Geometry: final body of the model. Coordinates: model frame, mm. Face numbers are marked on the shaded views. A direction names the side the tool comes from. Coordinates: 2 decimals unless noted, no trailing zeros. Loops run counter-clockwise (first coordinate to the right, second up) from the corner with the lowest first, then second, coordinate; pieces in that order, holes last. Notation, with made-up numbers: M 4.5,28 L 28.5,28 A32 ccw 28.5,55 Z; hole C 77,-28 d8. An arc over 180 degrees is marked long. Write each question's results on one line, items separated by ' | '. Start each with the question number.
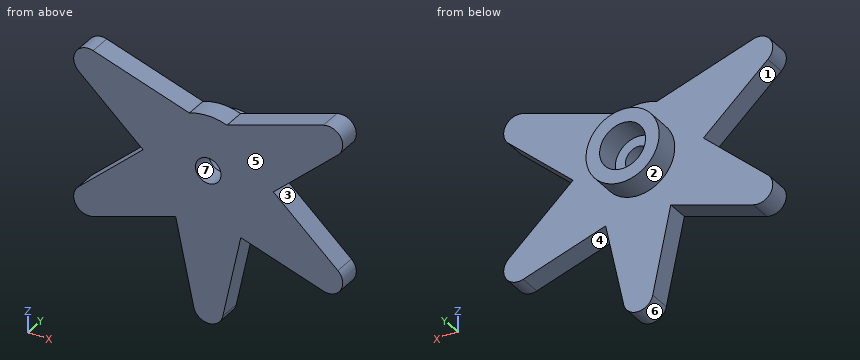
from build123d import *

# Parameters (mm, degrees)
SKETCH1_R           = 1.5
BOSS_EXTRUDE1_DEPTH = 2.6
SKETCH2_R           = 4.3
SKETCH2_R_2         = 2.7
BOSS_EXTRUDE2_DEPTH = 3


with BuildPart() as part:
    # Sketch1 → Boss-Extrude1 (new body)
    with BuildSketch(Plane(origin=(0, 0, 0), x_dir=(1, 0, 0), z_dir=(0, 1, 0))):
        with BuildLine():
            Line((3.832260045, 6.637669106), (1.711758301, 16.613845459))
            ThreePointArc((1.711758301, 16.613845459), (0, 18), (-1.711758301, 16.613845459))
            Line((-1.711758301, 16.613845459), (-3.832260045, 6.637669106))
            Line((-3.832260045, 6.637669106), (-13.532133071, 9.789348904))
            ThreePointArc((-13.532133071, 9.789348904), (-15.588457268, 9), (-15.243891373, 6.824496555))
            Line((-15.243891373, 6.824496555), (-7.664520091, 0))
            Line((-7.664520091, 0), (-15.243891373, -6.824496555))
            ThreePointArc((-15.243891373, -6.824496555), (-15.588457268, -9), (-13.532133071, -9.789348904))
            Line((-13.532133071, -9.789348904), (-2.213204152, -6.111605957))
            ThreePointArc((-2.213204152, -6.111605957), (0, -6.5), (2.213204152, -6.111605957))
            Line((2.213204152, -6.111605957), (13.532133071, -9.789348904))
            ThreePointArc((13.532133071, -9.789348904), (15.588457268, -9), (15.243891373, -6.824496555))
            Line((15.243891373, -6.824496555), (7.664520091, 0))
            Line((7.664520091, 0), (15.243891373, 6.824496555))
            ThreePointArc((15.243891373, 6.824496555), (15.588457268, 9), (13.532133071, 9.789348904))
            Line((13.532133071, 9.789348904), (3.832260045, 6.637669106))
        make_face()
        with Locations(Location((0, 0, 0), (0, 0, 270))):
            Circle(SKETCH1_R, mode=Mode.SUBTRACT)
    extrude(amount=BOSS_EXTRUDE1_DEPTH)

    # Sketch2 → Boss-Extrude2 (add)
    with BuildSketch(Plane(origin=(0, 2.6, 0), x_dir=(1, 0, 0), z_dir=(0, 1, 0))):
        with Locations(Location((0, 0, 0), (0, 0, 270))):
            Circle(SKETCH2_R)
        with Locations(Location((0, 0, 0), (0, 0, 270))):
            Circle(SKETCH2_R_2, mode=Mode.SUBTRACT)
    extrude(amount=BOSS_EXTRUDE2_DEPTH)


solid = part.part
Item 1: Set-up query: the marked faces 1, 2, 3 and 4. Return all of +Z, -Z, +X, -X, +Y, -Y with unobstructed straight access to the full face (end or side cutting, diameter ignored); none if empty.
Item 2: Section D-D, the plane y = 3.15. Return loops of the section in (x, z).
Item 3: Ray query, L1, parallel to X at y = 4.4, z = 0; L2, parallel to Y at x = 9.5, z = 5.25; L3, parallel to X at y = 1.45, z = -1. Return the intervals inside material, ascending. Write a range as [from, to].
Item 4: Contact query for a flat-ended pin moving along its axis: P1, Ø2.5, axis at x = 0.5, z = -0.5, coming from the +Y side. Output: stop coordinate, or through.
Item 5: Pull-direction query (X, two-part tool) for the marked faces 5, 6 and 7; classes: released by +X, released by -X, zero draft, split by the parting line, or undercut.
Item 6: Section B-B, the plane x = 0. Return loops of the section in (y, z), plus the area to 3 significant figures.
Item 7: Section C-C, the plane z = -1. Return loops of the section in (x, y), plus the area to 3 significant figures.
Solutions:
1) face 1: -X, +Y, -Y | face 2: +Y | face 3: +X, +Y, -Y | face 4: -Z, +Y, -Y
2) outline: C 0,0 d8.6; hole C 0,0 d5.4
3) L1: x = [-4.3, -2.7], [2.7, 4.3] | L2: y = [0, 2.6] | L3: x = [-8.78, -1.12], [1.12, 8.78]
4) P1: stops at y = 2.6
5) face 5: zero draft | face 6: split by the parting line | face 7: undercut
6) outline: M 0,-18 L 2.6,-18 L 2.6,-4.3 L 5.6,-4.3 L 5.6,-2.7 L 2.6,-2.7 L 2.6,-1.5 L 0,-1.5 Z; M 0,1.5 L 2.6,1.5 L 2.6,2.7 L 5.6,2.7 L 5.6,4.3 L 2.6,4.3 L 2.6,6.5 L 0,6.5 Z | area: 65.5 mm²
7) outline: M -8.78,0 L -1.12,0 L -1.12,2.6 L -2.51,2.6 L -2.51,5.6 L -4.18,5.6 L -4.18,2.6 L -8.78,2.6 Z; M 1.12,0 L 8.78,0 L 8.78,2.6 L 4.18,2.6 L 4.18,5.6 L 2.51,5.6 L 2.51,2.6 L 1.12,2.6 Z | area: 49.9 mm²
